Source: CAD feature listing. Evaluate the final solid. Frame: model axes, mm. Face numbers are marked on the shaded views. Round coordinates to 2 decimals unless told otherwise and drop trailing zeros. Loops run counter-clockwise (first coordinate to the right, second up) from the corner with the lowest first, then second, coordinate; pieces in that order, holes last. Notation, with made-up numbers: (81.5, 74) - (121.5, 74) arc R19 cw to (121.5, 82) - close; hole circle Ø2 at (0.5, -8.75). An arc over 180 degrees is marked (long way). One line per question, with ' | ' between items. Start each with the question number.
1. Cut plane C-C (x = 58). Return loops of the section in (y, z) (3 decimals), then the cut area to 3 significant figures.
2. Mould query, pull axis Z, two halves, no side actions, for the marked faces 1 and 2. Classes: pulls with the +Z half, pulls with the -Z half, needs draft (parallel to the pull), parting line crosses it, or undercut.
3. Pin query (flat end, axial travel): pin 1 (6 mm diameter, centred on x = -189.5, y = 20.5, fed in from +Z); pin 2 (3 mm diameter, centred on x = 347.5, y = 19.5, fed in from +Z); pin 3 (4 mm diameter, centred on x = 7.5, y = -39.5, fed in from -Z). Return the tip coordinate at first contact, or that it passes through.
4. Cut plane A-A (y = 0). Return loops of the section in (x, z) (3 decimals), then the cut area to 3 significant figures.
5. Ray query, line 1 (Y direction, x = -6, z = 0) (3 decimals); line 2 (Y direction, x = 176, z = -1.5); line 3 (Z direction, x = -59.5, y = 4.5). Return the intervals inside material, ascending.
```python
from build123d import *

# Parameters (mm, degrees)
SKETCH1_R           = 63.5
SKETCH1_R_2         = 60.325
BOSS_EXTRUDE1_DEPTH = 635
SKETCH3_R           = 66.675
BOSS_EXTRUDE3_DEPTH = 12.7
SKETCH13_R          = 60.325
CUT_EXTRUDE2_DEPTH  = 72.39


with BuildPart() as part:
    # Sketch1 → Boss-Extrude1 (new, symmetric)
    with BuildSketch(Plane(origin=(0, 0, 0), x_dir=(0, 0, -1), z_dir=(1, 0, 0))):
        with Locations(Location((0, 0, 0), (0, 0, 180))):
            Circle(SKETCH1_R)
        with Locations(Location((0, 0, 0), (0, 0, 180))):
            Circle(SKETCH1_R_2, mode=Mode.SUBTRACT)
    extrude(amount=BOSS_EXTRUDE1_DEPTH, both=True)

    # Sketch3 → Boss-Extrude3 (add, symmetric)
    with BuildSketch(Plane(origin=(0, 0, 0), x_dir=(0, 0, -1), z_dir=(1, 0, 0))):
        Circle(SKETCH3_R)
    extrude(amount=BOSS_EXTRUDE3_DEPTH, both=True)

    # Sketch13 → Cut-Extrude2 (cut, symmetric)
    with BuildSketch(Plane.ZY.offset(12.7)):
        Circle(SKETCH13_R)
    extrude(amount=CUT_EXTRUDE2_DEPTH, both=True, mode=Mode.SUBTRACT)


solid = part.part
```
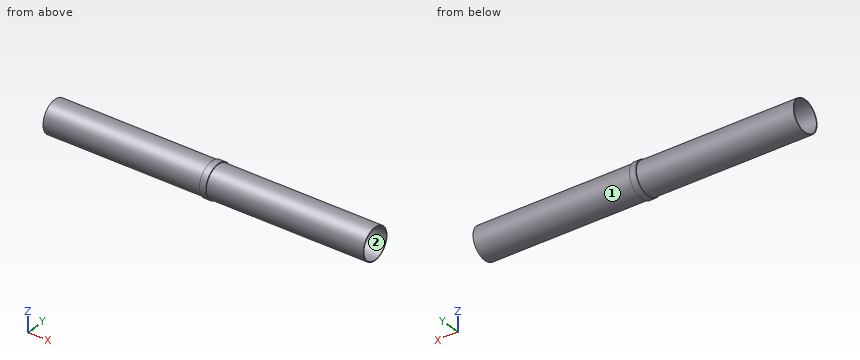
Answers follow:
1) outline: circle Ø127 at (0, 0); hole circle Ø120.65 at (0, 0) | area: 1,240 mm2
2) face 1: parting line crosses it | face 2: undercut
3) pin 1: stops at z = 61.04 | pin 2: stops at z = 60.9 | pin 3: stops at z = -55.13
4) outline: (-635, -63.5) - (-12.7, -63.5) - (-12.7, -66.675) - (12.7, -66.675) - (12.7, -63.5) - (635, -63.5) - (635, -60.325) - (-635, -60.325) - close; (-635, 60.325) - (635, 60.325) - (635, 63.5) - (12.7, 63.5) - (12.7, 66.675) - (-12.7, 66.675) - (-12.7, 63.5) - (-635, 63.5) - close | area: 8,230 mm2
5) line 1: y = -66.675 to -60.325, 60.325 to 66.675 | line 2: y = -63.48 to -60.31, 60.31 to 63.48 | line 3: z = -63.34 to -60.16, 60.16 to 63.34
